```python
from build123d import *

# Parameters (mm, degrees)
SKETCH_1_R      = 1.6
SKETCH_1_R_2    = 14.8
EXTRUDE_4_DEPTH = 4
SKETCH_1_6_W    = 22
SKETCH_1_6_H    = 8
SKETCH_1_6_R    = 1.6
EXTRUDE_5_DEPTH = 4
CHAMFER_1_SIZE  = 1.4
CHAMFER_2_SIZE  = 1
CHAMFER_3_SIZE  = 1
SKETCH_1_7_R    = 14.8
EXTRUDE_6_DEPTH = 9
SKETCH_2_R      = 15.8
EXTRUDE_7_DEPTH = 1


with BuildPart() as part:
    # 草图1 → 凸台-拉伸4 (new body)
    with BuildSketch(Plane(origin=(0, 0, 0), x_dir=(0, 0, -1), z_dir=(1, 0, 0))):
        with BuildLine():
            Line((23, -23.2), (23, 0))
            ThreePointArc((23, 0), (0, 23), (-23, 0))
            Line((-23, 0), (-23, -23.2))
            Line((-23, -23.2), (23, -23.2))
        make_face()
        with Locations((11.619884993, 15.420108208)):
            Circle(SKETCH_1_R, mode=Mode.SUBTRACT)
        with Locations((-11.619884993, -15.420108208)):
            Circle(SKETCH_1_R, mode=Mode.SUBTRACT)
        with Locations((15.420108208, -11.619884993)):
            Circle(SKETCH_1_R, mode=Mode.SUBTRACT)
        with Locations((-15.420108208, 11.619884993)):
            Circle(SKETCH_1_R, mode=Mode.SUBTRACT)
        Circle(SKETCH_1_R_2, mode=Mode.SUBTRACT)
    extrude(amount=EXTRUDE_4_DEPTH)

    # 草图1<6> → 凸台-拉伸5 (add)
    with BuildSketch(Plane(origin=(0, 0, 0), x_dir=(0, 0, -1), z_dir=(1, 0, 0))):
        with Locations((0, -27.2)):
            Rectangle(SKETCH_1_6_W, SKETCH_1_6_H)
        with Locations((-6, -27.2)):
            Circle(SKETCH_1_6_R, mode=Mode.SUBTRACT)
        with Locations((6, -27.2)):
            Circle(SKETCH_1_6_R, mode=Mode.SUBTRACT)
    extrude(amount=EXTRUDE_5_DEPTH)

    # 倒角1
    chamfer_1_edges = [part.edges().sort_by_distance(p)[0] for p in [
        (4, -15.420108208, 13.219884993),
        (4, -11.619884993, -13.820108208),
        (4, 15.420108208, -10.019884993),
        (4, 11.619884993, 17.020108208),
    ]]
    chamfer(chamfer_1_edges, length=CHAMFER_1_SIZE)

    # 倒角2
    chamfer_2_edges = [part.edges().sort_by_distance(p)[0] for p in [
        (4, -27.2, 7.6),
    ]]
    chamfer(chamfer_2_edges, length=CHAMFER_2_SIZE)

    # 倒角3
    chamfer_3_edges = [part.edges().sort_by_distance(p)[0] for p in [
        (4, -27.2, -4.4),
    ]]
    chamfer(chamfer_3_edges, length=CHAMFER_3_SIZE)

    # 草图1<7> → 凸台-拉伸6 (add)
    with BuildSketch(Plane(origin=(0, 0, 0), x_dir=(0, 0, -1), z_dir=(1, 0, 0))):
        Circle(SKETCH_1_7_R)
    extrude(amount=EXTRUDE_6_DEPTH)

    # 草图2 → 凸台-拉伸7 (add)
    with BuildSketch(Plane(origin=(4, 0, 0), x_dir=(0, 0, -1), z_dir=(1, 0, 0))):
        Circle(SKETCH_2_R)
    extrude(amount=EXTRUDE_7_DEPTH)


solid = part.part
```
Source: CAD feature listing. Evaluate the final solid. Frame: model axes, mm. A direction names the side the tool comes from. Give positions to 0.01 mm unless a question says otherwise; leave off trailing zeros. Order: outer loops, then holes, each group sorted by start corner. A loop starts at its lowest first (then second) coordinate and runs counter-clockwise, first axis right, second up.
(1) Section query D-D (x = 7.25). Return the cut outline in (y, z), plus the area to 3 significant figures.
(2) Section query C-C (z = 6). Return the cut outline in (x, y), plus the area to 3 significant figures.
(3) Contact query for flat-ended pins moving along their axis: P1, Ø4, axis at x = 4.5, y = 4.5, coming from the +Z side; P2, Ø2, axis at x = 2.5, y = -26, coming from the -Z side; P3, Ø1, axis at x = 3, z = 12.5, coming from the +Y side. Output: stop coordinate, or through.
(4) Pull-direction query (Z, two-part tool) for faces 4 (the face through (0, -4, 0)), 5 (the face through (1.28, 11.01, 13.94)), 6 (the face through (2, -27, -11)); classes: +Z half, -Z half, draft (parallel to the pull), parting line (faces both ways), or undercut.
(5) Material intervals for line 1 along Y through (x, z) = (1.25, 0); line 2 along Z through (x, y) = (4.5, 5.5); line 3 along X through (y, z) = (-23, -6.5), sorted ascending.
(6) Access query for faces 1 (the face through (2, -23.2, -17)), 2 (the face through (5, -12, -9)), 3 (the face through (2, -27, 11)). Directions: +Z, -Z, +X, -X, +Y, -Y. A direction counts if a zero-diameter tool reaches every point of the face in a straight line with its end or side. Return the directions, or none.
(7) Section query A-A (y = -27.2). Return the cut outline in (x, z).
(8) Section query B-B (z = 0). Return the cut outline in (x, y), plus the area to 3 significant figures.
Outcome:
1. outline: circle Ø29.6 at (0, 0)
1. area: 688 mm2
2. outline: (0, -31.2) - (4, -31.2) - (4, -29.8) - (3, -28.8) - (0, -28.8) - close; (0, -25.6) - (3, -25.6) - (4, -24.6) - (4, -14.62) - (5, -14.62) - (5, -13.53) - (9, -13.53) - (9, 13.53) - (5, 13.53) - (5, 14.62) - (4, 14.62) - (4, 22.2) - (0, 22.2) - close
2. area: 337 mm2
3. P1: stops at z = 22.86
3. P2: stops at z = -11
3. P3: stops at y = 19.62
4. face 4: draft
4. face 5: undercut
4. face 6: -Z half
5. line 1: y = -31.2 to 23
5. line 2: z = -14.81 to 14.81
5. line 3: x = 0 to 4
6. face 1: -Z, +X, -X, -Y
6. face 2: +X
6. face 3: +Z, +X, -X, -Y
7. outline: (0, -11) - (4, -11) - (4, -8.6) - (3, -7.6) - (0, -7.6) - close; (0, -4.4) - (3, -4.4) - (4, -3.4) - (4, 3.4) - (3, 4.4) - (0, 4.4) - close; (0, 7.6) - (3, 7.6) - (4, 8.6) - (4, 11) - (0, 11) - close
8. outline: (0, -31.2) - (4, -31.2) - (4, -15.8) - (5, -15.8) - (5, -14.8) - (9, -14.8) - (9, 14.8) - (5, 14.8) - (5, 15.8) - (4, 15.8) - (4, 23) - (0, 23) - close
8. area: 367 mm2
